The model under review builds one solid part; all positions refer to its coordinate system, in mm. A direction names the side the tool comes from. Round coordinates to 2 decimals unless told otherwise and drop trailing zeros. Write each loop counter-clockwise with the first axis right and the second up, starting at its lowest first coordinate (ties: lowest second). Pieces come first, ordered by that corner, then holes. Notation, with made-up numbers: (55, -23.75) - (112, -23.75) arc R18 ccw to (112, -3.75) - close; hole circle Ø10 at (39.5, -1.5). An arc over 180 degrees is marked (long way). Return JSON: item names as keys, results as strings.
from build123d import *

# Parameters (mm, degrees)
SKETCH1_W           = 30
SKETCH1_H           = 3
BOSS_EXTRUDE1_DEPTH = 5
BOSS_EXTRUDE3_DEPTH = 5
LPATTERN2_COUNT     = 9
LPATTERN2_PITCH     = 3.5


with BuildPart() as part:
    # Sketch1 → Boss-Extrude1 (new body)
    with BuildSketch(Plane(origin=(0, 0, 0), x_dir=(0, 0, -1), z_dir=(1, 0, 0))):
        Rectangle(SKETCH1_W, SKETCH1_H)
    extrude(amount=BOSS_EXTRUDE1_DEPTH)

    # Sketch2 → Boss-Extrude3 (add)
    with BuildSketch(Plane(origin=(5, 0, 0), x_dir=(0, 0, -1), z_dir=(1, 0, 0))):
        Polygon((15, 1.5), (13, 1.5), (18.641236999, 7.141236999), (19.358763001, 5.858763001), align=None)
    boss_extrude3 = extrude(amount=-BOSS_EXTRUDE3_DEPTH)

    # LPattern2: Boss-Extrude3 ×9
    with Locations(*[(0, 0, i * LPATTERN2_PITCH) for i in range(1, LPATTERN2_COUNT)]):
        add(boss_extrude3)


solid = part.part
(1) Clearance check with flat-ended pins moving along their axes: pin 1 Ø1.5 at (x, z) = (2, -6) entering from +Y; pin 2 Ø1.5 at (x, y) = (2, 0.5) entering from -Z; pin 3 Ø1.2 at (x, z) = (3.5, -2) entering from +Y; pin 4 Ø1 at (y, z) = (1.5, -10) entering from -X. State where each tip first meets the part, or that it passes through.
Filled in:
{"pin 1": "stops at y = 6.05", "pin 2": "stops at z = -15", "pin 3": "stops at y = 6.68", "pin 4": "stops at x = 0"}
(2) Add section A-A (z = -13.5). Write out the cut boundary in (x, y), plus the area to 3 significant figures.
Filled in:
{"outline": "(0, -1.5) - (5, -1.5) - (5, 2) - (0, 2) - close; (0, 3.5) - (5, 3.5) - (5, 5.5) - (0, 5.5) - close", "area": "27.5 mm2"}
(3) Wall thickness on line 1 (Y direction, x = 1.35, z = 12); line 2 (Z direction, x = 1.8, y = 0); line 3 (Y direction, x = 2.5, z = -11): over which ranges is each line inside the solid? List them lowest first.
Filled in:
{"line 1": "y = -1.5 to 1.5, 2.5 to 4.5", "line 2": "z = -15 to 15", "line 3": "y = -1.5 to 3, 4.5 to 6.5"}
(4) For faces 4 (the flat face through (2.5, 6.5, 2)), 5 (the flat face through (2.5, 3.7, 10.8)), 6 (the flat face through (2, -1.5, 0)), list the 3-axis set-ups (+Z, -Z, +X, -X, +Y, -Y) from which the entire face can be reached by the end or side of a thin tool; tool diameter is ignored.
Filled in:
{"face 4": "+X, -X, +Y", "face 5": "+X, -X", "face 6": "+Z, -Z, +X, -X, -Y"}
(5) Add section C-C (y = -0.5). Write out the cut boundary in (x, z), plus the area to 3 significant figures.
Filled in:
{"outline": "(0, -15) - (5, -15) - (5, 15) - (0, 15) - close", "area": "150 mm2"}
(6) Mouldability with a two-part tool opening along Z and no side actions: class faces 1 (the flat face through (2.5, 6.5, -8.5)), 2 (the flat face through (2, 0, -15)), 3 (the flat face through (5, 1, -2)) as released by +Z, released by -Z, zero draft, split by the parting line, or undercut.
Filled in:
{"face 1": "undercut", "face 2": "released by -Z", "face 3": "zero draft"}
(7) Add section B-B (y = 4.75). Give the number of separate pieces and of enclosed holes in the cut face, plus the area to 3 significant figures.
Filled in:
{"separate pieces": "9", "enclosed holes": "0", "area": "90.0 mm2"}
